For this review, take the finished solid that the model builds, in its own axes (mm). A direction names the side the tool comes from. Round coordinates to 2 decimals unless told otherwise and drop trailing zeros. Loops run counter-clockwise (first coordinate to the right, second up) from the corner with the lowest first, then second, coordinate; pieces in that order, holes last.
1. To check wall thickness, follow line 1 along Y through (x, z) = (1.05, 0); line 2 along Y through (x, z) = (1.8, 0); line 3 along Y through (x, z) = (3, 6.5). State the ranges of each line that lie inside material, in increasing order.
2. Consider section A-A on z = 0. State the section outline as (x, y) points (3 decimals).
3. Draft analysis for pull direction Y (two halves, no side actions). For faces 1 (the flat face through (3.175, 3, 3)), 2 (the cylindrical face through (1.565, 3.755, -11.923)), 3 (the cylindrical face through (2.29, 6.5, -10.36)), 4 (the cylindrical face through (0.697, -5.045, -9.194)), state which applies: released by +Y, released by -Y, zero draft, split by the parting line, or undercut.
4. Consider section C-C on z = 3. State the section outline as (x, y) points (3 decimals).
5. Clearance check with flat-ended pins moving along their axes: pin 1 Ø2 at (y, z) = (4.38, -7.58) entering from +X; pin 2 Ø4 at (y, z) = (-4.38, -7.58) entering from +X (3 decimals); pin 3 Ø1 at (x, z) = (0.5, -4.5) entering from +Y; pin 4 Ø1 at (x, y) = (1.5, 1.5) entering from -Z. State where each tip first meets the part, or that it passes through.
6. Tool access review of faces 5 (the cylindrical face through (0.697, 5.928, 8.385)), 6 (the cylindrical face through (2.288, -5.333, -0.759)): name each direction out of +Z, -Z, +X, -X, +Y, -Y from which nothing blocks a thin tool from reaching the whole face with its end or side.
7. Consider section D-D on x = 0.95. State the section outline as (y, z) points (3 decimals), then the cut area to 3 significant figures.
8. Consider section B-B on y = 0. State the section outline as (x, z) points (3 decimals), then the cut area to 3 significant figures.
from build123d import *

# Parameters (mm, degrees)
SKETCH1_R           = 12.5
BOSS_EXTRUDE1_DEPTH = 3.175
SKETCH3_R           = 4
CUT_EXTRUDE1_DEPTH  = 18.960529641
SKETCH2_R           = 1.75
CUT_EXTRUDE2_DEPTH  = 18.960529641
SKETCH4_R           = 3.5
SKETCH4_R_2         = 1.75
CUT_EXTRUDE3_DEPTH  = 1.8
CIRPATTERN1_COUNT   = 6


with BuildPart() as part:
    # Sketch1 → Boss-Extrude1 (new body)
    with BuildSketch(Plane(origin=(0, 0, 0), x_dir=(0, 0, -1), z_dir=(1, 0, 0))):
        Circle(SKETCH1_R)
    extrude(amount=BOSS_EXTRUDE1_DEPTH)

    # Sketch3 → Cut-Extrude1 (cut, through all)
    with BuildSketch(Plane(origin=(3.175, 0, 0), x_dir=(0, 0, -1), z_dir=(1, 0, 0))):
        Circle(SKETCH3_R)
    extrude(amount=-CUT_EXTRUDE1_DEPTH, mode=Mode.SUBTRACT)

    # Sketch2 → Cut-Extrude2 (cut, through all)
    with BuildSketch(Plane(origin=(3.175, 0, 0), x_dir=(0, 0, -1), z_dir=(1, 0, 0))):
        with Locations((0, 8.75)):
            Circle(SKETCH2_R)
    cut_extrude2 = extrude(amount=-CUT_EXTRUDE2_DEPTH, mode=Mode.SUBTRACT)

    # Sketch4 → Cut-Extrude3 (cut)
    # profile 1 of 3: a face of its own
    with BuildSketch(Plane(origin=(3.175, 0, 0), x_dir=(0, 0, -1), z_dir=(1, 0, 0))):
        with Locations((0, 8.75)):
            Circle(SKETCH4_R)
        Polygon((3.175426481, 8.75), (1.58771324, 11.5), (-1.58771324, 11.5), (-3.175426481, 8.75), (-1.58771324, 6), (1.58771324, 6), align=None, mode=Mode.SUBTRACT)
    # profile 2 of 3: a face of its own
    with BuildSketch(Plane(origin=(3.175, 0, 0), x_dir=(0, 0, -1), z_dir=(1, 0, 0))):
        Polygon((1.58771324, 6), (3.175426481, 8.75), (1.58771324, 11.5), (-1.58771324, 11.5), (-3.175426481, 8.75), (-1.58771324, 6), align=None)
        with Locations((0, 8.75)):
            Circle(SKETCH4_R_2, mode=Mode.SUBTRACT)
    # profile 3 of 3: a face of its own
    with BuildSketch(Plane(origin=(3.175, 0, 0), x_dir=(0, 0, -1), z_dir=(1, 0, 0))):
        with Locations((0, 8.75)):
            Circle(SKETCH4_R_2)
    cut_extrude3 = extrude(amount=-CUT_EXTRUDE3_DEPTH, mode=Mode.SUBTRACT)

    # CirPattern1: Cut-Extrude2, Cut-Extrude3 ×6 about axis
    cirpattern1_axis = Axis((0, 0, 0), (1, 0, 0))
    add([cut_extrude2.rotate(cirpattern1_axis, i * 360 / CIRPATTERN1_COUNT) for i in range(1, CIRPATTERN1_COUNT)], mode=Mode.SUBTRACT)
    add([cut_extrude3.rotate(cirpattern1_axis, i * 360 / CIRPATTERN1_COUNT) for i in range(1, CIRPATTERN1_COUNT)], mode=Mode.SUBTRACT)


solid = part.part
Resolved:
1. line 1: y = -12.5 to -10.5, -7 to -4, 4 to 7, 10.5 to 12.5
1. line 2: y = -12.5 to -12.25, -5.25 to -4, 4 to 5.25, 12.25 to 12.5
1. line 3: y = -10.68 to -7.7, -1.05 to 1.05, 7.7 to 10.68
2. outline: (0, -12.5) - (3.175, -12.5) - (3.175, -12.25) - (1.375, -12.25) - (1.375, -10.5) - (0, -10.5) - close; (0, -7) - (1.375, -7) - (1.375, -5.25) - (3.175, -5.25) - (3.175, -4) - (0, -4) - close; (0, 4) - (3.175, 4) - (3.175, 5.25) - (1.375, 5.25) - (1.375, 7) - (0, 7) - close; (0, 10.5) - (1.375, 10.5) - (1.375, 12.25) - (3.175, 12.25) - (3.175, 12.5) - (0, 12.5) - close
3. face 1: zero draft
3. face 2: split by the parting line
3. face 3: undercut
3. face 4: undercut
4. outline: (0, -12.135) - (3.175, -12.135) - (3.175, -10.553) - (1.375, -10.553) - (1.375, -6.947) - (3.175, -6.947) - (3.175, -2.646) - (0, -2.646) - close; (0, 2.646) - (3.175, 2.646) - (3.175, 6.947) - (1.375, 6.947) - (1.375, 10.553) - (3.175, 10.553) - (3.175, 12.135) - (0, 12.135) - close
5. pin 1: passes through
5. pin 2: stops at x = 1.375
5. pin 3: stops at y = 11.84
5. pin 4: stops at z = -12.46
6. face 5: +X, -X
6. face 6: +X
7. outline: circle Ø25 at (0, 0); hole circle Ø3.5 at (-8.75, 0); hole circle Ø3.5 at (-4.375, -7.578); hole circle Ø3.5 at (-4.375, 7.578); hole circle Ø8 at (0, 0); hole circle Ø3.5 at (4.375, -7.578); hole circle Ø3.5 at (4.375, 7.578); hole circle Ø3.5 at (8.75, 0)
7. area: 383 mm2
8. outline: (0, -12.5) - (3.175, -12.5) - (3.175, -4) - (0, -4) - close; (0, 4) - (3.175, 4) - (3.175, 12.5) - (0, 12.5) - close
8. area: 54.0 mm2
